from build123d import *

# Parameters (mm, degrees)
BOSS_EXTRUDE1_DEPTH = 490
FILLET1_R           = 100


with BuildPart() as part:
    # Sketch1 → Boss-Extrude1 (new body, symmetric)
    with BuildSketch(Plane.XY):
        Polygon((0, 1100), (0, 0), (350, 0), (350, 280), (200, 1100), align=None)
    extrude(amount=BOSS_EXTRUDE1_DEPTH, both=True)

    # Fillet1
    fillet1_edges = [part.edges().sort_by_distance(p)[0] for p in [
        (350, 140, 490),
        (275, 690, 490),
        (275, 690, -490),
        (350, 140, -490),
        (200, 1100, 0),
        (350, 0, 0),
    ]]
    fillet(fillet1_edges, radius=FILLET1_R)


solid = part.part
CAD build for the part. Positions are in the model's coordinates, mm. Give positions to 0.01 mm unless a question says otherwise; leave off trailing zeros. Order: outer loops, then holes, each group sorted by start corner. A loop starts at its lowest first (then second) coordinate and runs counter-clockwise, first axis right, second up. Notation, with made-up numbers: (-27, -16.5) - (4, -16.5) arc R26 cw to (4, 16.5) - close; hole circle Ø6 at (70.5, 46.5). An arc over 180 degrees is marked (long way). Write each question's results on one line, items separated by ' | '.
1. Saw through at B-B on z = -404. List the corners of the cut face in (x, y).
Calculated:
outline: (0, 0) - (250, 0) arc R100 ccw to (349.02, 86) - (349.02, 279.91) - (211.51, 1031.59) arc R100 ccw to (116.63, 1100) - (0, 1100) - close
2. Probe L1, parallel to X at y = 270, z = -394.5; L2, parallel to X at y = 94.5, z = 105; L3, parallel to Z at x = 298, y = 263. List the from-to ranges inside material, lowest first. Write a range as from..to.
Calculated:
L1: x = 0..349.9 | L2: x = 0..349.85 | L3: z = -477.73..477.73
3. Pin check, flat tips, straight feed: pin 1 (3 mm diameter, centred on y = 824, z = -219, fed in from +X); pin 2 (8 mm diameter, centred on x = 224.5, y = 829, fed in from -Z). Stop position of each tip, or through.
Calculated:
pin 1: stops at x = 250.76 | pin 2: stops at z = -460.08
4. Saw through at A-A on z = 112.5. List the corners of the cut face in (x, y), and give its area (3 significant figures).
Calculated:
outline: (0, 0) - (250, 0) arc R100 ccw to (350, 100) - (350, 280) - (215, 1017.99) arc R100 ccw to (116.63, 1100) - (0, 1100) - close | area: 320,000 mm2
